Geometry: final body of the model. Coordinates: model frame, mm. Face numbers are marked on the shaded views. A direction names the side the tool comes from. Give positions to 0.01 mm unless a question says otherwise; leave off trailing zeros. Order: outer loops, then holes, each group sorted by start corner. A loop starts at its lowest first (then second) coordinate and runs counter-clockwise, first axis right, second up. Notation, with made-up numbers: (74.5, 44.5) - (116.5, 44.5) arc R19 cw to (116.5, 49.5) - close; hole circle Ø7 at (70, 26.5). An arc over 180 degrees is marked (long way). One line per item, written item: value.
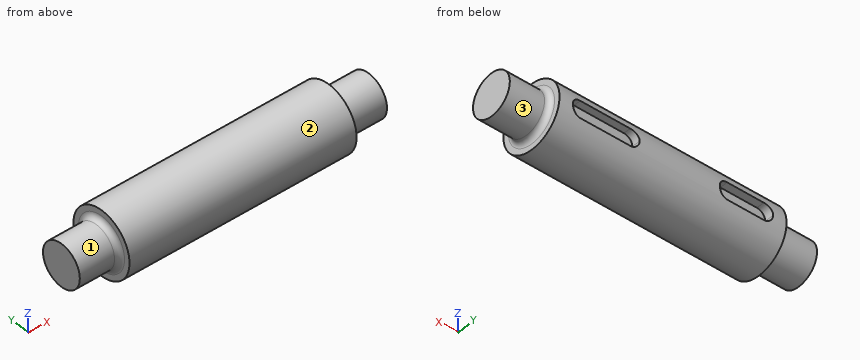
```python
from build123d import *

# Parameters (mm, degrees)
SKETCH1_R                = 20
BOSS_EXTRUDE1_DEPTH      = 38.1
SKETCH2_R                = 30.48
BOSS_EXTRUDE2_DEPTH      = 215.9
SKETCH3_R                = 19.9999981
BOSS_EXTRUDE3_DEPTH      = 38.1
FILLET1_R                = 5.08
SKETCH6_W                = 16.002
SKETCH6_H                = 16.002
CUT_EXTRUDE1_DEPTH       = 50.8
SKETCH7_W                = 16
SKETCH7_H                = 16
CUT_EXTRUDE2_DEPTH       = 63.5
BOSS_EXTRUDE4_REACH      = 300.305
BOSS_EXTRUDE4_END_RADIUS = 30.48
BOSS_EXTRUDE5_REACH      = 300.423
BOSS_EXTRUDE5_END_RADIUS = 30.48


with BuildPart() as part:
    # Sketch1 → Boss-Extrude1 (new body)
    with BuildSketch(Plane(origin=(0, 0, 0), x_dir=(0, 0, -1), z_dir=(1, 0, 0))):
        with Locations(Location((0, 0, 0), (0, 0, 180))):
            Circle(SKETCH1_R)
    extrude(amount=BOSS_EXTRUDE1_DEPTH)

    # Sketch2 → Boss-Extrude2 (add)
    with BuildSketch(Plane(origin=(38.1, 0, 0), x_dir=(0, 0, -1), z_dir=(1, 0, 0))):
        Circle(SKETCH2_R)
    extrude(amount=BOSS_EXTRUDE2_DEPTH)

    # Sketch3 → Boss-Extrude3 (add)
    with BuildSketch(Plane(origin=(254, 0, 0), x_dir=(0, 0, -1), z_dir=(1, 0, 0))):
        with Locations(Location((0, 0, 0), (0, 0, 180))):
            Circle(SKETCH3_R)
    extrude(amount=BOSS_EXTRUDE3_DEPTH)

    # Fillet1
    fillet1_edges = [part.edges().sort_by_distance(p)[0] for p in [
        (38.1, 0, -20),
        (254, 0, -19.9999981),
    ]]
    fillet(fillet1_edges, radius=FILLET1_R)

    # Sketch6 → Cut-Extrude1 (cut)
    with BuildSketch(Plane(origin=(50.8, 0, 0), x_dir=(0, 0, -1), z_dir=(1, 0, 0))):
        with Locations((0, 29.812996)):
            Rectangle(SKETCH6_W, SKETCH6_H)
    extrude(amount=CUT_EXTRUDE1_DEPTH, mode=Mode.SUBTRACT)

    # Sketch7 → Cut-Extrude2 (cut)
    with BuildSketch(Plane.ZY.offset(-177.8)):
        with Locations((0, 30.48)):
            Rectangle(SKETCH7_W, SKETCH7_H)
    extrude(amount=-CUT_EXTRUDE2_DEPTH, mode=Mode.SUBTRACT)

    # Boss-Extrude4: up to this cylinder (the profile starts inside it)
    boss_extrude4_end = Plane(origin=(76.2, 0, 0), z_dir=(-1, 0, 0)) * Cylinder(BOSS_EXTRUDE4_END_RADIUS, 709.795666, mode=Mode.PRIVATE)
    # Sketch8 → Boss-Extrude4 (add, up to the surface)
    with BuildSketch(Plane(origin=(0, 21.811996, 0), x_dir=(1, 0, 0), z_dir=(0, 1, 0)), mode=Mode.PRIVATE) as boss_extrude4_sk1:
        with BuildLine():
            Line((58.801, 8.001), (50.8, 8.001))
            Line((50.8, 8.001), (50.8, 0))
            ThreePointArc((50.8, 0), (53.143438644, 5.657561356), (58.801, 8.001))
        make_face()
    boss_extrude4_tool1 = extrude(boss_extrude4_sk1.sketch, amount=BOSS_EXTRUDE4_REACH, mode=Mode.PRIVATE) & boss_extrude4_end
    add(boss_extrude4_tool1.solids().sort_by_distance((52.587167, 21.811996, -6.213833))[0])
    # Sketch8 → Boss-Extrude4 (add, up to the surface)
    with BuildSketch(Plane(origin=(0, 21.811996, 0), x_dir=(1, 0, 0), z_dir=(0, 1, 0)), mode=Mode.PRIVATE) as boss_extrude4_sk2:
        with BuildLine():
            ThreePointArc((58.801, -8.001), (53.143438644, -5.657561356), (50.8, 0))
            Line((50.8, 0), (50.8, -8.001))
            Line((50.8, -8.001), (58.801, -8.001))
        make_face()
    boss_extrude4_tool2 = extrude(boss_extrude4_sk2.sketch, amount=BOSS_EXTRUDE4_REACH, mode=Mode.PRIVATE) & boss_extrude4_end
    add(boss_extrude4_tool2.solids().sort_by_distance((52.587167, 21.811996, 6.213833))[0])
    # Sketch8 → Boss-Extrude4 (add, up to the surface)
    with BuildSketch(Plane(origin=(0, 21.811996, 0), x_dir=(1, 0, 0), z_dir=(0, 1, 0)), mode=Mode.PRIVATE) as boss_extrude4_sk3:
        with BuildLine():
            ThreePointArc((101.6, 0), (99.256561356, -5.657561356), (93.599, -8.001))
            Line((93.599, -8.001), (101.6, -8.001))
            Line((101.6, -8.001), (101.6, 0))
        make_face()
    boss_extrude4_tool3 = extrude(boss_extrude4_sk3.sketch, amount=BOSS_EXTRUDE4_REACH, mode=Mode.PRIVATE) & boss_extrude4_end
    add(boss_extrude4_tool3.solids().sort_by_distance((99.812833, 21.811996, 6.213833))[0])
    # Sketch8 → Boss-Extrude4 (add, up to the surface)
    with BuildSketch(Plane(origin=(0, 21.811996, 0), x_dir=(1, 0, 0), z_dir=(0, 1, 0)), mode=Mode.PRIVATE) as boss_extrude4_sk4:
        with BuildLine():
            Line((101.6, 8.001), (93.599, 8.001))
            ThreePointArc((93.599, 8.001), (99.256561356, 5.657561356), (101.6, 0))
            Line((101.6, 0), (101.6, 8.001))
        make_face()
    boss_extrude4_tool4 = extrude(boss_extrude4_sk4.sketch, amount=BOSS_EXTRUDE4_REACH, mode=Mode.PRIVATE) & boss_extrude4_end
    add(boss_extrude4_tool4.solids().sort_by_distance((99.812833, 21.811996, -6.213833))[0])

    # Boss-Extrude5: up to this cylinder (the profile starts inside it)
    boss_extrude5_end = Plane(origin=(209.55, 0, 0), z_dir=(-1, 0, 0)) * Cylinder(BOSS_EXTRUDE5_END_RADIUS, 722.732112, mode=Mode.PRIVATE)
    # Sketch10 → Boss-Extrude5 (add, up to the surface)
    with BuildSketch(Plane(origin=(0, 22.48, 0), x_dir=(1, 0, 0), z_dir=(0, 1, 0)), mode=Mode.PRIVATE) as boss_extrude5_sk1:
        with BuildLine():
            ThreePointArc((177.8, 0), (180.143145751, 5.656854249), (185.8, 8))
            Line((185.8, 8), (177.8, 8))
            Line((177.8, 8), (177.8, 0))
        make_face()
    boss_extrude5_tool1 = extrude(boss_extrude5_sk1.sketch, amount=BOSS_EXTRUDE5_REACH, mode=Mode.PRIVATE) & boss_extrude5_end
    add(boss_extrude5_tool1.solids().sort_by_distance((179.586944, 22.48, -6.213056))[0])
    # Sketch10 → Boss-Extrude5 (add, up to the surface)
    with BuildSketch(Plane(origin=(0, 22.48, 0), x_dir=(1, 0, 0), z_dir=(0, 1, 0)), mode=Mode.PRIVATE) as boss_extrude5_sk2:
        with BuildLine():
            ThreePointArc((185.8, -8), (180.143145751, -5.656854249), (177.8, 0))
            Line((177.8, 0), (177.8, -8))
            Line((177.8, -8), (185.8, -8))
        make_face()
    boss_extrude5_tool2 = extrude(boss_extrude5_sk2.sketch, amount=BOSS_EXTRUDE5_REACH, mode=Mode.PRIVATE) & boss_extrude5_end
    add(boss_extrude5_tool2.solids().sort_by_distance((179.586944, 22.48, 6.213056))[0])
    # Sketch10 → Boss-Extrude5 (add, up to the surface)
    with BuildSketch(Plane(origin=(0, 22.48, 0), x_dir=(1, 0, 0), z_dir=(0, 1, 0)), mode=Mode.PRIVATE) as boss_extrude5_sk3:
        with BuildLine():
            Line((241.3, -8), (241.3, 0))
            ThreePointArc((241.3, 0), (238.956854249, -5.656854249), (233.3, -8))
            Line((233.3, -8), (241.3, -8))
        make_face()
    boss_extrude5_tool3 = extrude(boss_extrude5_sk3.sketch, amount=BOSS_EXTRUDE5_REACH, mode=Mode.PRIVATE) & boss_extrude5_end
    add(boss_extrude5_tool3.solids().sort_by_distance((239.513056, 22.48, 6.213056))[0])
    # Sketch10 → Boss-Extrude5 (add, up to the surface)
    with BuildSketch(Plane(origin=(0, 22.48, 0), x_dir=(1, 0, 0), z_dir=(0, 1, 0)), mode=Mode.PRIVATE) as boss_extrude5_sk4:
        with BuildLine():
            Line((241.3, 8), (233.3, 8))
            ThreePointArc((233.3, 8), (238.956854249, 5.656854249), (241.3, 0))
            Line((241.3, 0), (241.3, 8))
        make_face()
    boss_extrude5_tool4 = extrude(boss_extrude5_sk4.sketch, amount=BOSS_EXTRUDE5_REACH, mode=Mode.PRIVATE) & boss_extrude5_end
    add(boss_extrude5_tool4.solids().sort_by_distance((239.513056, 22.48, -6.213056))[0])


solid = part.part
```
1) Material intervals for line 1 along X through (y, z) = (-26.5, -3); line 2 along Z through (x, y) = (140, -21.5); line 3 along X through (y, z) = (-22, -1), sorted ascending.
Answers below:
line 1: 38.1 to 254
line 2: -21.61 to 21.61
line 3: 37.08 to 255.02
2) Section B-B, the plane x = 264. Return loops of the section in (y, z), then the cut area to 3 significant figures.
Answers below:
outline: circle Ø40 at (0, 0)
area: 1,260 mm^2
3) Set-up query: the marked faces 1, 2 and 3. Return all of +Z, -Z, +X, -X, +Y, -Y with unobstructed straight access to the full face (end or side cutting, diameter ignored); none if empty.
Answers below:
face 1: -X
face 2: +X, -X
face 3: +X
4) First-contact query: pin 1 (8 mm diameter, centred on y = 0, z = 1.5, fed in from -X); pin 2 (8 mm diameter, centred on x = 121.5, z = 12.5, fed in from -Y); pin 3 (2 mm diameter, centred on x = 218, y = 27, fed in from +Z); pin 4 (6 mm diameter, centred on x = 79, y = 25.5, fed in from -Z). Flat tips, straight axial feed; report the tip coordinate or a pass-through.
Answers below:
pin 1: x = 0
pin 2: y = -29.27
pin 3: z = 15.91
pin 4: z = -20.56
5) Section C-C, the plane x = 220. Return loops of the section in (y, z), then the cut area to 3 significant figures.
Answers below:
outline: (22.48, -8) - (22.48, 8) - (29.41, 8) arc R30.48 ccw (long way) to (29.41, -8) - close
area: 2,800 mm^2
6) Section A-A, the plane y = 0. Return loops of the section in (x, z).
Answers below:
outline: (0, -20) - (33.02, -20) arc R5.08 cw to (38.1, -25.08) - (38.1, -30.48) - (254, -30.48) - (254, -25.08) arc R5.08 cw to (259.08, -20) - (292.1, -20) - (292.1, 20) - (259.08, 20) arc R5.08 cw to (254, 25.08) - (254, 30.48) - (38.1, 30.48) - (38.1, 25.08) arc R5.08 cw to (33.02, 20) - (0, 20) - close
7) Section D-D, the plane x = 126. Return loops of the section in (y, z).
Answers below:
outline: circle Ø60.96 at (0, 0)
